For this review, use the dimensioned drawing (mm, ordinates from the lowest corner) and the shaded views. A direction names the side the tool comes from. Give positions to 0.01 mm unless a question says otherwise; leave off trailing zeros. Order: outer loops, then holes, each group sorted by start corner. A loop starts at its lowest first (then second) coordinate and runs counter-clockwise, first axis right, second up. Notation, with made-up numbers: M 70,-1.5 L 105,-1.5 A25 ccw 105,36.5 Z; hole C 25.25,72.5 d6. An arc over 180 degrees is marked long. Answer as CSV lines item,"result". Start each with the question number.
1. Clearance check with flat-ended pins moving along their axes: P1, Ø8, axis at x = 115, y = 633.5, coming from the -Z side; P2, Ø1.5, axis at x = 79, z = 1038, coming from the +Y side. State where each tip first meets the part, or that it passes through.
2. We need section C-C, the plane z = 622.5. Give the boundary of the cut face in (x, y), and give its area (3 significant figures).
3. Machinability: for the marked faces 1 and 2, which of the approach directions +Z, -Z, +X, -X, +Y, -Y give a long, thin tool a straight path to every point of the face, cutting with its end or side? Answer none if there is none.
4. Mouldability with a two-part tool opening along Z and no side actions: class the marked faces 3, 4, 5 and 6 as pulls with the +Z half, pulls with the -Z half, needs draft (parallel to the pull), parting line crosses it, or undercut.
5. For line 1 along Z through (x, y) = (44, 103); line 2 along Z through (x, y) = (115.5, 399); line 3 along Y through (x, z) = (113.5, 608), list the stretches that pass through material, from the lowest coordinate up.
6. We need section B-B, the plane x = 51. Give the boundary of the cut face in (y, z).
7. We need section D-D, the plane y = 563. Give the boundary of the cut face in (x, z).
8. We need section A-A, the plane y = 207. Give the boundary of the cut face in (x, z).
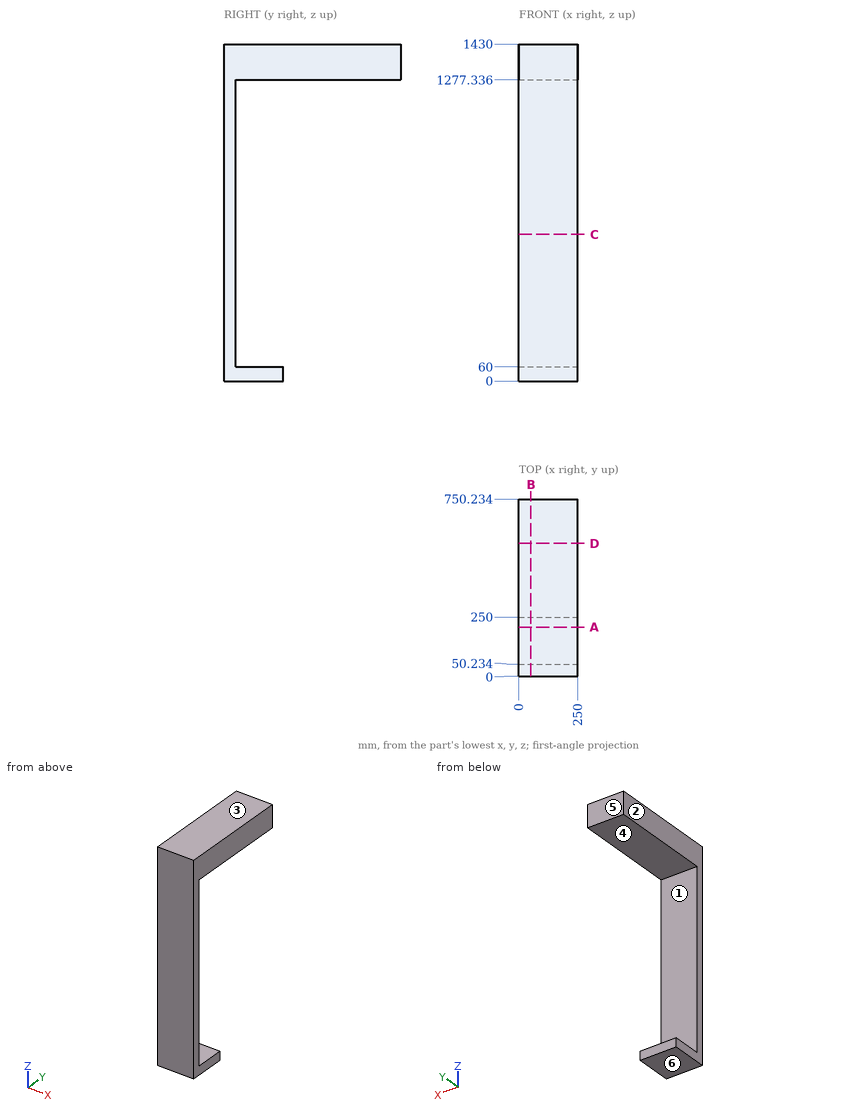
Result set:
1,P1,"z = 1277.34"
1,P2,"y = 50.23"
2,outline,"M 0,0 L 250,0 L 250,50.23 L 0,50.23 Z"
2,area,"12,600 mm2"
3,face 1,"+X, -X, +Y"
3,face 2,"+Z, -Z, -X, +Y, -Y"
4,face 3,"pulls with the +Z half"
4,face 4,"undercut"
4,face 5,"needs draft"
4,face 6,"pulls with the -Z half"
5,line 1,"0 to 60, 1277.34 to 1430"
5,line 2,"1277.34 to 1430"
5,line 3,"0 to 50.23"
6,outline,"M 0,0 L 250,0 L 250,60 L 50.23,60 L 50.23,1277.34 L 750.23,1277.34 L 750.23,1430 L 0,1430 Z"
7,outline,"M 0,1277.34 L 250,1277.34 L 250,1430 L 0,1430 Z"
8,outline,"M 0,0 L 250,0 L 250,60 L 0,60 Z; M 0,1277.34 L 250,1277.34 L 250,1430 L 0,1430 Z"
